from build123d import *

# Parameters (mm, degrees)
BOSS_EXTRUDE2_DEPTH                       = 162.814
CUT_EXTRUDE1_DEPTH                        = 166.821138692
SKETCH6_W                                 = 6.35
SKETCH6_H                                 = 6.1722
SKETCH6_H_2                               = 6.35
CUT_EXTRUDE2_DEPTH                        = 166.821138692
CSK_FOR_6_FLAT_HEAD_MACHINE_SCREW_2_COUNT = 2
CSK_FOR_6_FLAT_HEAD_MACHINE_SCREW_2_PITCH = 123.248406325


with BuildPart() as part:
    # Sketch3 → Boss-Extrude2 (new body)
    with BuildSketch(Plane(origin=(0, 0, 0), x_dir=(0, 0, -1), z_dir=(1, 0, 0))):
        Polygon((-0.5715, 31.420044321), (-1.5875, 30.833456448), (-1.5875, -1.917455679), (-0.5715, -1.330867805), align=None)
    extrude(amount=BOSS_EXTRUDE2_DEPTH)

    # Sketch5 → Cut-Extrude1 (cut, through all)
    with BuildSketch(Plane.XY.offset(1.5875)):
        Polygon((0, -1.917455679), (16.672349491, 31.420044321), (0, 31.420044321), align=None)
        Polygon((162.814, -1.917455679), (146.141650509, 31.420044321), (162.814, 31.420044321), align=None)
    extrude(amount=-CUT_EXTRUDE1_DEPTH, mode=Mode.SUBTRACT)

    # Sketch6 → Cut-Extrude2 (cut, through all)
    with BuildSketch(Plane.XY.offset(1.5875)):
        with Locations((19.880593675, 11.641857216)):
            Rectangle(SKETCH6_W, SKETCH6_H)
        with Locations((143.129, 11.641857216)):
            Rectangle(SKETCH6_W, SKETCH6_H)
        with Locations((81.593696837, 11.552957216)):
            Rectangle(SKETCH6_W, SKETCH6_H_2)
    extrude(amount=-CUT_EXTRUDE2_DEPTH, mode=Mode.SUBTRACT)

    # Sketch7 → CSK for #6 Flat Head Machine Screw (100)1 (revolve, cut)
    with BuildSketch(Plane(origin=(19.939, 19.426957216, 1.5875), x_dir=(0, -1, 0), z_dir=(1, 0, 0))):
        Polygon((0, 0), (0, 1.016), (1.89865, 1.016), (1.89865, 1.380025208), (3.5433, 0), align=None)
    csk_for_6_flat_head_machine_screw_100 = revolve(axis=Axis((19.939, 19.426957216, 7.9375), (0, 0, -1)), mode=Mode.SUBTRACT)

    # CSK for _6 Flat Head Machine Screw _ 2: CSK for #6 Flat Head Machine Screw (100)1 ×2
    with Locations(*[(i * CSK_FOR_6_FLAT_HEAD_MACHINE_SCREW_2_PITCH, 0, 0) for i in range(1, CSK_FOR_6_FLAT_HEAD_MACHINE_SCREW_2_COUNT)]):
        add(csk_for_6_flat_head_machine_screw_100, mode=Mode.SUBTRACT)


solid = part.part
Work out the finished part from the listing and answer in its coordinate system (mm). Coordinates: 2 decimals unless noted, no trailing zeros. Write each loop counter-clockwise with the first axis right and the second up, starting at its lowest first coordinate (ties: lowest second). Pieces come first, ordered by that corner, then holes. Notation, with made-up numbers: M 15,41 L 54,41 A17 cw 54,62 Z; hole C -8,-7.5 d3. An arc over 180 degrees is marked long. Write item = value, one per line.
1. Flat-ended cylindrical pins translate along their axes: pin 1 (0.5 mm diameter, centred on y = 10, z = 1.5, fed in from -X) (3 decimals); pin 2 (0.5 mm diameter, centred on y = 12, z = 1, fed in from +X). Find the tip coordinate at first contact, or state that the pin passes through.
Solution:
pin_1 = 5.835
pin_2 = 155.98
2. The part is cut by section D-D (y = 21.5). State how many separate pieces and enclosed holes the cut face has, then the cut area to 3 significant figures.
Solution:
separate_pieces = 3
enclosed_holes = 0
area = 133 mm2
3. The part is cut by section B-B (y = 13). Determine the outline of the cut face in (x, z).
Solution:
outline = M 7.46,0.57 L 16.71,0.57 L 16.71,1.59 L 7.46,1.59 Z; M 23.06,0.57 L 78.42,0.57 L 78.42,1.59 L 23.06,1.59 Z; M 84.77,0.57 L 139.95,0.57 L 139.95,1.59 L 84.77,1.59 Z; M 146.3,0.57 L 155.35,0.57 L 155.35,1.59 L 146.3,1.59 Z
4. Determine the mould class of faces 1 (the face through (80, 18, 1.588)), 2 (the face through (154.595, 14.518, 1.087)), 3 (the face through (8.22, 14.52, 1.09)) for opening direction X: released by +X, released by -X, zero draft, split by the parting line, or undercut.
Solution:
face_1 = zero draft
face_2 = released by +X
face_3 = released by -X
5. The part is cut by section C-C (x = 118.5). Determine the outline of the cut face in (y, z), then the cut area to 3 significant figures.
Solution:
outline = M -1.92,1.59 L -1.33,0.57 L 31.42,0.57 L 30.83,1.59 Z
area = 33.3 mm2
6. The part is cut by section A-A (z = 1.2). Determine the outline of the cut face in (x, y).
Solution:
outline = M 0.11,-1.69 L 162.7,-1.69 L 146.32,31.06 L 16.49,31.06 Z; hole M 16.71,8.56 L 23.06,8.56 L 23.06,14.73 L 16.71,14.73 Z; hole C 19.94,19.43 d6.16; hole M 78.42,8.38 L 84.77,8.38 L 84.77,14.73 L 78.42,14.73 Z; hole M 139.95,8.56 L 146.3,8.56 L 146.3,14.73 L 139.95,14.73 Z; hole C 143.19,19.43 d6.16
7. Straight lines are drawn through the part: line 1 (X direction, y = 18, z = 0.9); line 2 (X direction, y = 9.5, z = 1.3); line 3 (X direction, y = 11.5, z = 1.2). For each, find the intervals that lie inside material, in ascending order. Write a range as from..to.
Solution:
line_1 = 9.96..17.62, 22.26..140.87, 145.51..152.85
line_2 = 5.71..16.71, 23.06..78.42, 84.77..139.95, 146.3..157.1
line_3 = 6.71..16.71, 23.06..78.42, 84.77..139.95, 146.3..156.1
